from build123d import *

# Parameters (mm, degrees)
CROQUIS1_W              = 10
CROQUIS1_H              = 3
SALIENTE_EXTRUIR1_DEPTH = 3
REDONDEO1_R             = 10
CROQUIS2_W              = 6
CROQUIS2_H              = 3
CORTAR_EXTRUIR1_DEPTH   = 3
CROQUIS3_W              = 1.25
CROQUIS3_H              = 2.5
CROQUIS3_W_2            = 3
CROQUIS3_H_2            = 7.5
CROQUIS3_H_3            = 2
CORTAR_EXTRUIR2_DEPTH   = 32.032241298
CROQUIS4_W              = 3
CROQUIS4_H              = 5
CROQUIS4_W_2            = 4
CORTAR_EXTRUIR3_DEPTH   = 32.032241298
CROQUIS5_W              = 3
CROQUIS5_H              = 7.5
CROQUIS5_H_2            = 2.5
CROQUIS5_W_2            = 1.25
CROQUIS5_H_3            = 2
CORTAR_EXTRUIR4_DEPTH   = 32.032241298


with BuildPart() as part:
    # Croquis1 → Saliente-Extruir1 (new body)
    with BuildSketch(Plane.XY):
        Polygon((15, -17), (15, -24), (-15, -24), (-15, -19), (-5, -1.679491924), (-5, 24), (10, 24), (10, -8.339745962), align=None)
        with Locations((-10, -25.5)):
            Rectangle(CROQUIS1_W, CROQUIS1_H)
        with Locations((10, -25.5)):
            Rectangle(CROQUIS1_W, CROQUIS1_H)
    extrude(amount=SALIENTE_EXTRUIR1_DEPTH)

    # Redondeo1
    redondeo1_edges = [part.edges().sort_by_distance(p)[0] for p in [
        (-15, -19, 1.5),
        (-5, -1.679491924, 1.5),
        (10, -8.339745962, 1.5),
        (15, -17, 1.5),
    ]]
    fillet(redondeo1_edges, radius=REDONDEO1_R)

    # Croquis2 → Cortar-Extruir1 (cut)
    with BuildSketch(Plane.XY):
        with Locations((2.5, 22.5)):
            Rectangle(CROQUIS2_W, CROQUIS2_H)
    extrude(amount=CORTAR_EXTRUIR1_DEPTH, mode=Mode.SUBTRACT)

    # Croquis3 → Cortar-Extruir2 (cut, through all)
    with BuildSketch(Plane.XY):
        with Locations((0.375, 15.25)):
            Rectangle(CROQUIS3_W, CROQUIS3_H)
        with Locations((2.5, 15.25)):
            Rectangle(CROQUIS3_W_2, CROQUIS3_H)
        with Locations((4.625, 15.25)):
            Rectangle(CROQUIS3_W, CROQUIS3_H)
        with Locations((2.5, 20.25)):
            Rectangle(CROQUIS3_W_2, CROQUIS3_H_2)
        with Locations((2.5, 13)):
            Rectangle(CROQUIS3_W_2, CROQUIS3_H_3)
    extrude(amount=CORTAR_EXTRUIR2_DEPTH, mode=Mode.SUBTRACT)

    # Croquis4 → Cortar-Extruir3 (cut, through all)
    with BuildSketch(Plane.XY):
        with Locations((-3.5, 17.5)):
            Rectangle(CROQUIS4_W, CROQUIS4_H)
        with Locations((-4, 2.5)):
            Rectangle(CROQUIS4_W_2, CROQUIS4_H)
    extrude(amount=CORTAR_EXTRUIR3_DEPTH, mode=Mode.SUBTRACT)

    # Croquis5 → Cortar-Extruir4 (cut, through all)
    with BuildSketch(Plane.XY):
        with Locations((0, -23.25)):
            Rectangle(CROQUIS5_W, CROQUIS5_H)
        with Locations((0, -18.25)):
            Rectangle(CROQUIS5_W, CROQUIS5_H_2)
        with Locations((-2.125, -18.25)):
            Rectangle(CROQUIS5_W_2, CROQUIS5_H_2)
        with Locations((2.125, -18.25)):
            Rectangle(CROQUIS5_W_2, CROQUIS5_H_2)
        with Locations((0, -16)):
            Rectangle(CROQUIS5_W, CROQUIS5_H_3)
    extrude(amount=CORTAR_EXTRUIR4_DEPTH, mode=Mode.SUBTRACT)


solid = part.part
The listing builds one solid part. Answer for the finished solid, in the listing's coordinates (mm). A direction names the side the tool comes from. Give positions to 0.01 mm unless a question says otherwise; leave off trailing zeros. Write each loop counter-clockwise with the first axis right and the second up, starting at its lowest first coordinate (ties: lowest second). Pieces come first, ordered by that corner, then holes. Notation, with made-up numbers: (-30, 50) -> (-9, 50) arc R20 ccw to (-9, 62) -> close; hole circle Ø9 at (-8.75, 55.25). An arc over 180 degrees is marked (long way). Use a Markdown table: item, result.
(1) Find the intervals of material crossed by probe 1 along Y at (x, z) = (-3.5, 0.6); probe 2 along X at (y, z) = (22.5, 1.3); probe 3 along Y at (x, z) = (2.5, 0.65), in increasing order. Write a range as from..to.
Return value:
| item | result |
|---|---|
| probe 1 | -24..0, 5..15, 20..24 |
| probe 2 | -5..-0.5, 5.5..10 |
| probe 3 | -24..-19.5, -17..12 |
(2) Section A-A, the plane y = 17 is taken. Determine the outline of the cut face in (x, z).
Return value:
| item | result |
|---|---|
| outline | (-2, 0) -> (1, 0) -> (1, 3) -> (-2, 3) -> close; (4, 0) -> (10, 0) -> (10, 3) -> (4, 3) -> close |
(3) Section C-C, the plane x = 3.25 is taken. Determine the outline of the cut face in (y, z).
Return value:
| item | result |
|---|---|
| outline | (-24, 0) -> (12, 0) -> (12, 3) -> (-24, 3) -> close |
(4) Flat-ended cylindrical pins translate along their axes: P1, Ø1.5, axis at y = 18, z = 2, coming from the -X side; P2, Ø0.9, axis at y = 8.5, z = 1.5, coming from the -X side; P3, Ø0.9, axis at y = 6.5, z = 2, coming from the +X side; P4, Ø3, axis at x = 10.5, y = -8.5, coming from the +Z side. Find the tip coordinate at first contact, or state that the pin passes through.
Return value:
| item | result |
|---|---|
| P1 | x = -2 |
| P2 | x = -5 |
| P3 | x = 10 |
| P4 | z = 3 |
(5) Section B-B, the plane y = -23 is taken. Determine the outline of the cut face in (x, z), then the cut area to 3 significant figures.
Return value:
| item | result |
|---|---|
| outline | (-15, 0) -> (-1.5, 0) -> (-1.5, 3) -> (-15, 3) -> close; (1.5, 0) -> (15, 0) -> (15, 3) -> (1.5, 3) -> close |
| area | 81.0 mm2 |
(6) Section D-D, the plane y = 7 is taken. Determine the outline of the cut face in (x, z).
Return value:
| item | result |
|---|---|
| outline | (-5, 0) -> (10, 0) -> (10, 3) -> (-5, 3) -> close |
(7) For faces 1 (the flat face through (5, 21, 1)), 2 (the flat face through (-10, -27, 1)), 3 (the flat face through (-4, 5, 1)), 4 (the flat face through (0, 16.5, 1)), 5 (the flat face through (1.5, -16, 1)), determine the directions among +Z, -Z, +X, -X, +Y, -Y from which every point of the face is accessible in a straight line to the end or side of a thin tool.
Return value:
| item | result |
|---|---|
| face 1 | +Z, -Z, +Y |
| face 2 | +Z, -Z, +X, -X, -Y |
| face 3 | +Z, -Z, -X |
| face 4 | +Z, -Z |
| face 5 | +Z, -Z, -Y |
